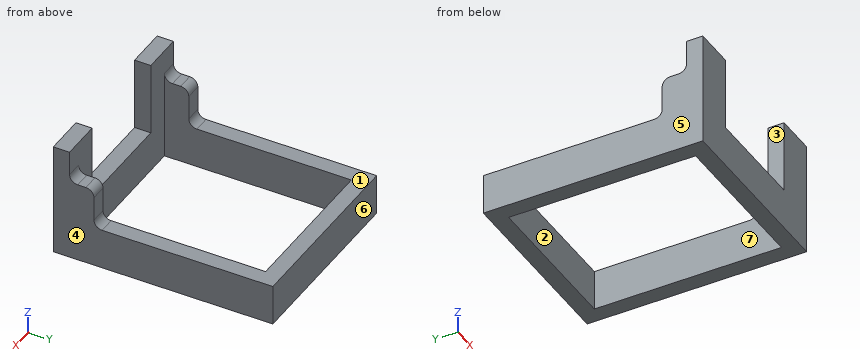
from build123d import *

# Parameters (mm, degrees)
F0_W     = 23
F0_H     = 27
F0_W_2   = 19
F0_H_2   = 23
F1_DEPTH = 5
F3_DEPTH = 5
F5_DEPTH = 5
F7_DEPTH = 4
F8_W     = 5
F8_H     = 2
F9_DEPTH = 4
F10_R    = 1


with BuildPart() as f1:
    # F0 (on Top) → F1 (new body)
    with BuildSketch(Plane.XY):
        with Locations((9.5, 11.5)):
            Rectangle(F0_W, F0_H)
        with Locations((9.5, 11.5)):
            Rectangle(F0_W_2, F0_H_2, mode=Mode.SUBTRACT)
    extrude(amount=F1_DEPTH)

    # F2 (on face) → F3 (join)
    with BuildSketch(Plane.XY.offset(5)):
        Polygon((3, 0), (0, 0), (0, 3), (-2, 3), (-2, -2), (3, -2), align=None)
    extrude(amount=F3_DEPTH)

    # F4 (on face) → F5 (join)
    with BuildSketch(Plane.XY.offset(5)):
        Polygon((19, 3), (19, 0), (16, 0), (16, -2), (21, -2), (21, 3), align=None)
    extrude(amount=F5_DEPTH)

    # F6 (on face) → F7 (join)
    with BuildSketch(Plane.XY.offset(10)):
        Polygon((3, 0), (0, 0), (-2, 0), (-2, -2), (3, -2), align=None)
    extrude(amount=F7_DEPTH)

    # F8 (on face) → F9 (join)
    with BuildSketch(Plane.XY.offset(10)):
        with Locations((18.5, -1)):
            Rectangle(F8_W, F8_H)
    extrude(amount=F9_DEPTH)

    # F10
    f10_edges = [f1.edges().sort_by_distance(p)[0] for p in [
        (20, 3, 5),
        (20, 0, 10),
        (20, 3, 10),
        (-1, 0, 10),
        (-1, 3, 10),
        (-1, 3, 5),
    ]]
    fillet(f10_edges, radius=F10_R)


solid = f1.part
Model file for the job. Use its own axes, mm. Face numbers are marked on the shaded views. A direction names the side the tool comes from. Coordinates: 2 decimals unless noted, no trailing zeros. Write each loop counter-clockwise with the first axis right and the second up, starting at its lowest first coordinate (ties: lowest second). Pieces come first, ordered by that corner, then holes. Notation, with made-up numbers: (64, 34) -> (105, 34) arc R10 cw to (105, 38) -> close; hole circle Ø4 at (44.5, 43.5). An arc over 180 degrees is marked (long way). One line per item, written item: value. Start each with the question number.
1) Pull direction X, two halves, no side cores. Call the marked faces 4, 5, 6 and 7: +X half, -X half, draft (parallel to the pull), parting line (faces both ways), or undercut.
2) Probe probe 1 along X at (y, z) = (15, 1.75); probe 2 along Y at (x, z) = (3, 2); probe 3 along Z at (x, y) = (19.5, 14.25). List the from-to ranges inside material, lowest first.
3) Slice it at A-A on z = 8. Write the cut outline in (x, y), then the cut area to 3 significant figures.
4) Slice it at B-B on x = 3.5. Write the cut outline in (y, z).
5) Flat gauge pins, fed straight in: pin 1 Ø8 at (x, y) = (8.5, 2) entering from +Z; pin 2 Ø2 at (x, z) = (20, 7) entering from +Y; pin 3 Ø0.5 at (x, y) = (20.5, 1.5) entering from +Z. Where does each tip first touch, or does it go through?
6) Slice it at C-C on y = 20. Write the cut outline in (x, z), then the cut area to 3 significant figures.
7) Which spindle directions (+Z, -Z, +X, -X, +Y, -Y) get a long thin tool onto all of the face, cutting with end or side? Do the marked faces 1, 2 and 3. Say none if no direction does.
8) Slice it at D-D on z = 2.5. Write the cut outline in (x, y).
Answers follow:
1. face 4: +X half
1. face 5: -X half
1. face 6: draft
1. face 7: undercut
2. probe 1: -2 to 0, 19 to 21
2. probe 2: -2 to 0, 23 to 25
2. probe 3: 0 to 5
3. outline: (-2, -2) -> (3, -2) -> (3, 0) -> (0, 0) -> (0, 3) -> (-2, 3) -> close; (16, -2) -> (21, -2) -> (21, 3) -> (19, 3) -> (19, 0) -> (16, 0) -> close
3. area: 32.0 mm2
4. outline: (-2, 0) -> (0, 0) -> (0, 5) -> (-2, 5) -> close; (23, 0) -> (25, 0) -> (25, 5) -> (23, 5) -> close
5. pin 1: z = 5
5. pin 2: y = 3
5. pin 3: z = 10
6. outline: (-2, 0) -> (0, 0) -> (0, 5) -> (-2, 5) -> close; (19, 0) -> (21, 0) -> (21, 5) -> (19, 5) -> close
6. area: 20.0 mm2
7. face 1: +Z, +X, -X, +Y
7. face 2: +Z, -Z
7. face 3: +Z, +Y, -Y
8. outline: (-2, -2) -> (21, -2) -> (21, 25) -> (-2, 25) -> close; hole (0, 0) -> (19, 0) -> (19, 23) -> (0, 23) -> close
